```python
from build123d import *

# Parameters (mm, degrees)
SKETCH1_R           = 14.6431
BOSS_EXTRUDE1_DEPTH = 7.366
FILLET1_SIZE        = 1.524
SHELL1_T            = 1.016
SKETCH2_W           = 5.08
SKETCH2_H           = 3.048
CUT_EXTRUDE1_DEPTH  = 25.4
FILLET2_R           = 0.381
SNAP_START          = 14.621716272
SNAP_GROOVE1_DEPTH  = 0.567483728
CIRPATTERN2_COUNT   = 4
FILLET3_R           = 2.54
FILLET4_R           = 2.54


# Read off the part's stored shape, not the designer's step: Snap Groove1
with BuildPart() as part:
    # Sketch1 → Boss-Extrude1 (new body)
    with BuildSketch(Plane(origin=(0, 0, 0), x_dir=(1, 0, 0), z_dir=(0, 1, 0))):
        with Locations(Location((0, 0, 0), (0, 0, 270))):
            Circle(SKETCH1_R)
    extrude(amount=BOSS_EXTRUDE1_DEPTH)

    # Fillet1
    fillet1_edges = [part.edges().sort_by_distance(p)[0] for p in [
        (0, 7.366, -14.6431),
    ]]
    chamfer(fillet1_edges, length=FILLET1_SIZE)

    # Shell1
    shell1_openings = [part.faces().sort_by_distance(p)[0] for p in [
        (0, 0, 0),
    ]]
    offset(amount=SHELL1_T, openings=shell1_openings, kind=Kind.INTERSECTION)

    # Sketch2 → Cut-Extrude1 (cut)
    with BuildSketch(Plane.XY):
        with Locations((0, 1.524)):
            Rectangle(SKETCH2_W, SKETCH2_H)
    extrude(amount=-CUT_EXTRUDE1_DEPTH, mode=Mode.SUBTRACT)

    # Fillet2
    fillet2_edges = [part.edges().sort_by_distance(p)[0] for p in [
        (15.607170203, 0, 1.274225676),
    ]]
    fillet(fillet2_edges, radius=FILLET2_R)

    # Snap Groove1 outline → Snap Groove1 (cut)
    with BuildSketch(Plane.XY.offset(SNAP_START)):
        Polygon((-0.707206527, 5.6642), (-0.791069456, 4.064), (0.791069456, 4.064), (0.707206527, 5.6642), align=None)
    snap_groove1 = extrude(amount=SNAP_GROOVE1_DEPTH, mode=Mode.SUBTRACT)

    # CirPattern2: Snap Groove1 ×4 about axis
    cirpattern2_axis = Axis((0, 0, 0), (0, 1, 0))
    for i in range(1, CIRPATTERN2_COUNT):
        add(snap_groove1.rotate(cirpattern2_axis, i * 360 / CIRPATTERN2_COUNT), mode=Mode.SUBTRACT)

    # Fillet3
    fillet3_edges = [part.edges().sort_by_distance(p)[0] for p in [
        (0, 8.382, -13.539940979),
    ]]
    fillet(fillet3_edges, radius=FILLET3_R)

    # Fillet4
    fillet4_edges = [part.edges().sort_by_distance(p)[0] for p in [
        (0, 6.262840979, -15.6591),
    ]]
    fillet(fillet4_edges, radius=FILLET4_R)


solid = part.part
```
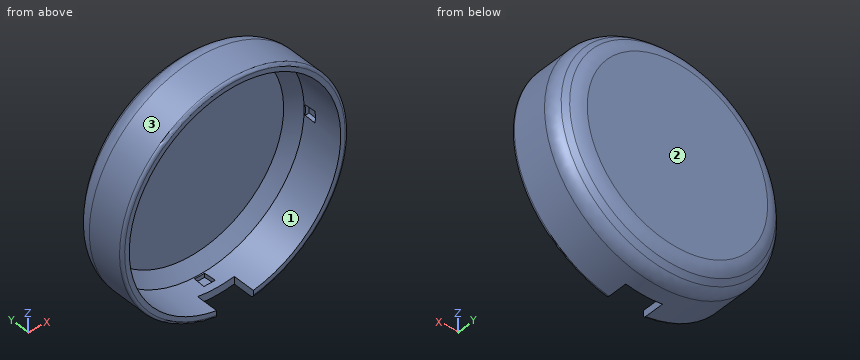
Work out the finished part from the listing and answer in its coordinate system (mm). Face numbers are marked on the shaded views. Give positions to 0.01 mm unless a question says otherwise; leave off trailing zeros. Loops run counter-clockwise (first coordinate to the right, second up) from the corner with the lowest first, then second, coordinate; pieces in that order, holes last. Notation, with made-up numbers: (82, -40) - (135, -40) arc R8 cw to (135, -36) - close; hole circle Ø10 at (59, 53.5). An arc over 180 degrees is marked (long way). Use CSV: the item, a comma, the result in double quotes. Start each with the question number.
(1) Each of these flat-tipped pins is pushed along its axis until it touches: pin 1 (5 mm diameter, centred on y = 1, z = 11, fed in from -X); pin 2 (4 mm diameter, centred on y = 2.5, z = -6.5, fed in from +X); pin 3 (1.5 mm diameter, centred on x = 8.5, z = 10, fed in from -Y). Where does it stop, or does it pass through?
(2) Find the intervals of material crossed by L1, parallel to X at y = 2.9, z = 0; L2, parallel to Z at x = 0, y = 4.2, in increasing order.
(3) Find section A-A, the plane y = 3.5. Determine the outline of the cut face in (x, z).
(4) Determine the mould class of the marked faces 1, 2 and 3 for opening direction X: released by +X, released by -X, zero draft, split by the parting line, or undercut.
Results found:
1,pin 1,"x = -13.15"
1,pin 2,"x = 15"
1,pin 3,"y = 6.61"
2,L1,"-15.66 to -14.64, 14.64 to 15.66"
2,L2,"-15.66 to -15.19, 15.19 to 15.66"
3,outline,"circle Ø31.32 at (0, 0); hole circle Ø29.29 at (0, 0)"
4,face 1,"undercut"
4,face 2,"zero draft"
4,face 3,"split by the parting line"
